Input: part model. Units: mm. Frame: model coordinates. A direction names the side the tool comes from. Coordinates: 2 decimals unless noted, no trailing zeros. Loops run counter-clockwise (first coordinate to the right, second up) from the corner with the lowest first, then second, coordinate; pieces in that order, holes last.
(1) Contact query for flat-ended pins moving along their axis: P1, Ø4, axis at x = 16.5, z = 13.5, coming from the +Y side; P2, Ø4.5, axis at x = 27, y = 30.5, coming from the +Z side; P3, Ø20, axis at x = 22.5, y = 14, coming from the -Z side; P4, Ø4, axis at y = 14, z = 15, coming from the +X side. Output: stop coordinate, or through.
(2) Mould query, pull axis X, two halves, no side actions, for faces 6 (the face through (32.661, 9.787, 12.395)), 7 (the face through (0, 14, 12)), 8 (the face through (23, 32, 6)), 9 (the face through (45, 14, 12)). Classes: released by +X, released by -X, zero draft, split by the parting line, or undercut.
(3) Set-up query: faces 1 (the face through (23, -4, 6)), 2 (the face through (33, 18, 5)), 3 (the face through (40.944, 11.918, 15.273)), 4 (the face through (22, 0, 14)), 5 (the face through (23, 30, 8)). Return all of +Z, -Z, +X, -X, +Y, -Y with unobstructed straight access to the full face (end or side cutting, diameter ignored); none if empty.
(4) Section D-D, the plane x = 5.5. Return loops of the section in (y, z).
(5) Section A-A, the plane x = 22.5. Return loops of the section in (y, z).
(6) Section B-B, the plane y = 18. Return loops of the section in (x, z).
(7) Section C-C, the plane z = 18.75. Return loops of the section in (x, y), then the cut area to 3 significant figures.
(8) Line query: L1, parallel to X at y = 14, z = 12.5; L2, parallel to Y at x = 22.5, z = 12.5; L3, parallel to Y at x = 40.5, z = 15. Output: solid intervals per line, ascending.
```python
from build123d import *

# Parameters (mm, degrees)
SKETCH1_W                 = 45
SKETCH1_H                 = 28
SKETCH1_R                 = 11
BOSS_EXTRUDE1_DEPTH       = 20
M5X0_8_TAPPED_HOLE1_D     = 4.2
M5X0_8_TAPPED_HOLE1_DEPTH = 8
M5X0_8_TAPPED_HOLE1_TIP   = 1.2618073
SKETCH6_W                 = 45
SKETCH6_H                 = 28
CUT_EXTRUDE1_DEPTH        = 5
SKETCH7_W                 = 45
SKETCH7_H                 = 4
BOSS_EXTRUDE5_DEPTH       = 3


with BuildPart() as part:
    # Sketch1 → Boss-Extrude1 (new body)
    with BuildSketch(Plane.XY):
        with Locations((22.5, 14)):
            Rectangle(SKETCH1_W, SKETCH1_H)
        with Locations((22.5, 14)):
            Circle(SKETCH1_R, mode=Mode.SUBTRACT)
    extrude(amount=BOSS_EXTRUDE1_DEPTH)

    # M5x0.8 Tapped Hole1
    with Locations(Plane(origin=(45, 14, 15), x_dir=(0, 0, 1), z_dir=(1, 0, 0))):
        with Locations((0, 0)):
            Hole(M5X0_8_TAPPED_HOLE1_D / 2, depth=M5X0_8_TAPPED_HOLE1_DEPTH)
            with Locations((0, 0, -(M5X0_8_TAPPED_HOLE1_DEPTH + M5X0_8_TAPPED_HOLE1_TIP / 2))):  # 118° drill point
                Cone(0, M5X0_8_TAPPED_HOLE1_D / 2, M5X0_8_TAPPED_HOLE1_TIP, mode=Mode.SUBTRACT)

    # Sketch6 → Cut-Extrude1 (cut)
    with BuildSketch(Plane(origin=(0, 0, 0), x_dir=(-1, 0, 0), z_dir=(0, 0, -1))):
        with Locations((-22.5, 14)):
            Rectangle(SKETCH6_W, SKETCH6_H)
    extrude(amount=-CUT_EXTRUDE1_DEPTH, mode=Mode.SUBTRACT)

    # Sketch7 → Boss-Extrude5 (add)
    with BuildSketch(Plane(origin=(0, 0, 5), x_dir=(-1, 0, 0), z_dir=(0, 0, -1))):
        with Locations((-22.5, 30)):
            Rectangle(SKETCH7_W, SKETCH7_H)
        with Locations((-22.5, -2)):
            Rectangle(SKETCH7_W, SKETCH7_H)
    extrude(amount=-BOSS_EXTRUDE5_DEPTH)


solid = part.part
```
Report:
1. P1: stops at y = 28
1. P2: stops at z = 8
1. P3: passes through
1. P4: stops at x = 36.94
2. face 6: undercut
2. face 7: released by -X
2. face 8: zero draft
2. face 9: released by +X
3. face 1: +Z, -Z, +X, -X, -Y
3. face 2: -Z, +X, -X, +Y, -Y
3. face 3: +X
3. face 4: +Z, +X, -X, -Y
3. face 5: +Z, +X, -X, +Y
4. outline: (-4, 5) - (32, 5) - (32, 8) - (28, 8) - (28, 20) - (0, 20) - (0, 8) - (-4, 8) - close
5. outline: (-4, 5) - (3, 5) - (3, 20) - (0, 20) - (0, 8) - (-4, 8) - close; (25, 5) - (32, 5) - (32, 8) - (28, 8) - (28, 20) - (25, 20) - close
6. outline: (0, 5) - (12.25, 5) - (12.25, 20) - (0, 20) - close; (32.75, 5) - (45, 5) - (45, 20) - (32.75, 20) - close
7. outline: (0, 0) - (45, 0) - (45, 28) - (0, 28) - close; hole circle Ø22 at (22.5, 14)
7. area: 880 mm2
8. L1: x = 0 to 11.5, 33.5 to 45
8. L2: y = 0 to 3, 25 to 28
8. L3: y = 0 to 11.9, 16.1 to 28
